Build history of the part. All positions in model axes, mm. Face numbers are marked on the shaded views. A direction names the side the tool comes from. Give positions to 0.01 mm unless a question says otherwise; leave off trailing zeros. Order: outer loops, then holes, each group sorted by start corner. A loop starts at its lowest first (then second) coordinate and runs counter-clockwise, first axis right, second up. Notation, with made-up numbers: (50.5, 84) - (104.5, 84) arc R7 cw to (104.5, 91) - close; hole circle Ø5 at (3, -11.5). An arc over 180 degrees is marked (long way). Use a Markdown table: item, result. Add a question column.
(1) Slice it at B-B (y = 0). Write the cut outline in (x, z) (1 decimal).
(2) Slice it at A-A (x = 0). Write the cut outline in (y, z) (1 decimal).
(3) Slice it at D-D (x = -4). Write the cut outline in (y, z).
(4) Which spindle directions (+Z, -Z, +X, -X, +Y, -Y) get a long thin tool onto all of the face, cutting with end or side? Do the marked faces 5, 6 and 7. Say none if no direction does.
(5) Slice it at C-C (z = -5). Write the cut outline in (x, y) (1 decimal).
(6) Wall check: line 1 (Y direction, x = 0, z = -3); line 2 (Y direction, x = 0, z = 3.75) (3 decimals). Give the ranges that are in metal, low to high.
(7) Mould opens along Z. For the marked faces 1, 2, 3 and 4 say: +Z half, -Z half, draft (parallel to the pull), parting line (faces both ways), or undercut.
(8) Flat gauge pins, fed straight in: pin 1 (6 mm diameter, centred on y = -2.5, z = -2, fed in from +X); pin 2 (6 mm diameter, centred on x = -3.5, z = -4, fed in from -Y); pin 3 (2 mm diameter, centred on y = 2.5, z = -2.5, fed in from -X). Where does each tip first touch, or does it go through?
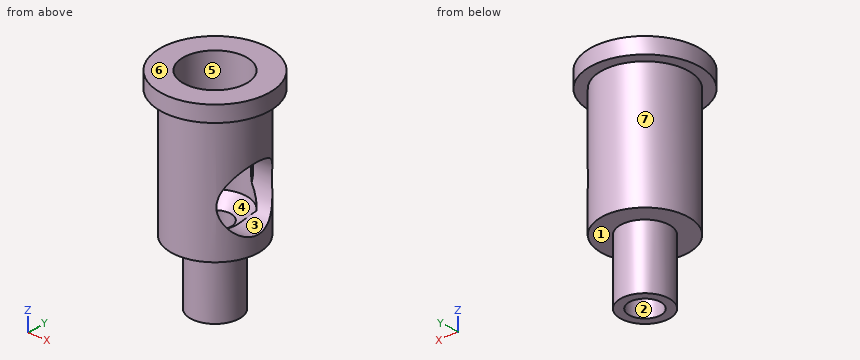
from build123d import *

# Parameters (mm, degrees)
F0_R      = 4.3688
F1_DEPTH  = 12.7
F2_R      = 5.461
F2_R_2    = 4.3688
F3_DEPTH  = 1.6002
F5_D      = 6.35
F5_DEPTH  = 12.065
F5_TIP    = 1.9077324654
F6_R      = 2.4511
F7_DEPTH  = 6.4008
F8_R      = 1.5875
F9_DEPTH  = 20.702
F12_D     = 6.35
F12_DEPTH = 3.302
F12_TIP   = 1.9077324654


with BuildPart() as f1:
    # F0 (on Top) → F1 (new body)
    with BuildSketch(Plane.XY):
        Circle(F0_R)
    extrude(amount=F1_DEPTH)

    # F2 (on face) → F3 (join)
    with BuildSketch(Plane.XY.offset(12.7)):
        Circle(F2_R)
        Circle(F2_R_2, mode=Mode.SUBTRACT)
        Circle(F2_R_2)
    extrude(amount=F3_DEPTH)

    # F5
    with Locations(Plane.XY.offset(14.3002)):
        with Locations((0, 0)):
            Hole(F5_D / 2, depth=F5_DEPTH)
            with Locations((0, 0, -(F5_DEPTH + F5_TIP / 2))):  # 118° drill point
                Cone(0, F5_D / 2, F5_TIP, mode=Mode.SUBTRACT)

    # F6 (on face) → F7 (join)
    with BuildSketch(Plane(origin=(0, 0, 0), x_dir=(1, 0, 0), z_dir=(0, 0, -1))):
        Circle(F6_R)
    extrude(amount=F7_DEPTH)

    # F8 (on face) → F9 (cut, through all)
    with BuildSketch(Plane(origin=(0, 0, -6.4008), x_dir=(1, 0, 0), z_dir=(0, 0, -1))):
        Circle(F8_R)
    extrude(amount=-F9_DEPTH, mode=Mode.SUBTRACT)

    # F12
    with Locations(Plane.YZ.offset(4.3688)):
        with Locations((0, 4.7752)):
            Hole(F12_D / 2, depth=F12_DEPTH)
            with Locations((0, 0, -(F12_DEPTH + F12_TIP / 2))):  # 118° drill point
                Cone(0, F12_D / 2, F12_TIP, mode=Mode.SUBTRACT)


solid = f1.part
Solution:
| question | item | result |
|---|---|---|
| 1 | outline | (-5.5, 12.7) - (-4.4, 12.7) - (-4.4, 0) - (-2.5, 0) - (-2.5, -6.4) - (-1.6, -6.4) - (-1.6, 1.3) - (-3.2, 2.2) - (-3.2, 14.3) - (-5.5, 14.3) - close; (1.6, -6.4) - (2.5, -6.4) - (2.5, 0) - (4.4, 0) - (4.4, 1.6) - (2.1, 1.6) - (1.6, 1.3) - close; (3.2, 8) - (4.4, 8) - (4.4, 12.7) - (5.5, 12.7) - (5.5, 14.3) - (3.2, 14.3) - close |
| 2 | outline | (-5.5, 12.7) - (-4.4, 12.7) - (-4.4, 0) - (-2.5, 0) - (-2.5, -6.4) - (-1.6, -6.4) - (-1.6, 1.3) - (-3.2, 2.2) - (-3.2, 14.3) - (-5.5, 14.3) - close; (1.6, -6.4) - (2.5, -6.4) - (2.5, 0) - (4.4, 0) - (4.4, 12.7) - (5.5, 12.7) - (5.5, 14.3) - (3.2, 14.3) - (3.2, 2.2) - (1.6, 1.3) - close |
| 3 | outline | (-3.72, 12.7) - (-1.76, 12.7) - (-1.76, 0) - (1.76, 0) - (1.76, 12.7) - (3.72, 12.7) - (3.72, 14.3) - (-3.72, 14.3) - close |
| 4 | face 5 | +Z |
| 4 | face 6 | +Z, +X, -X, +Y, -Y |
| 4 | face 7 | -Z |
| 5 | outline | circle Ø4.9 at (0, 0); hole circle Ø3.2 at (0, 0) |
| 6 | line 1 | -2.45 to -1.59, 1.59 to 2.45 |
| 6 | line 2 | -4.369 to -3.175, 3.175 to 4.369 |
| 7 | face 1 | -Z half |
| 7 | face 2 | draft |
| 7 | face 3 | undercut |
| 7 | face 4 | +Z half |
| 8 | pin 1 | x = 4.36 |
| 8 | pin 2 | y = -2.4 |
| 8 | pin 3 | x = -1.94 |
